Could you check a few things on this model? Use its own coordinates, in mm. Face numbers are marked on the shaded views. A direction names the side the tool comes from. Give positions to 0.01 mm unless a question says otherwise; leave off trailing zeros. Write each loop counter-clockwise with the first axis right and the second up, starting at its lowest first coordinate (ties: lowest second). Pieces come first, ordered by that corner, then holes. Notation, with made-up numbers: M -35.75,-24 L -16.75,-24 A18 cw -16.75,-11 Z; hole C 54.5,12 d2. An arc over 180 degrees is marked long. One line per item, written item: value.
```python
from build123d import *

# Parameters (mm, degrees)
F0_R      = 38.84
F0_R_2    = 27.5
F1_DEPTH  = 10.14
F2_R      = 41.875
F3_DEPTH  = 4.57
F4_R      = 41.875
F6_R      = 40.925
F8_R      = 40
F9_DEPTH  = 8.65
F10_R     = 41.95
F11_DEPTH = 13.57
F12_R     = 39.7
F13_DEPTH = 11.49
F14_R     = 31
F15_DEPTH = 16.29
F16_R     = 27.295707
F17_DEPTH = 2.75
F18_R     = 29.375
F19_DEPTH = 6
F20_R     = 28.5
F21_DEPTH = 1.3
F22_R     = 27.25
F23_DEPTH = 5.5
F24_R     = 28.475
F25_DEPTH = 12.25


with BuildPart() as f1:
    # F0 (on Front) → F1 (new body)
    with BuildSketch(Plane.XZ):
        Circle(F0_R)
        Circle(F0_R_2, mode=Mode.SUBTRACT)
    extrude(amount=F1_DEPTH)

    # F2 (on face) → F3 (join)
    with BuildSketch(Plane.XZ.offset(10.14)):
        Circle(F2_R)
    extrude(amount=F3_DEPTH)

    # F4 (on face) → F7 section 0
    with BuildSketch(Plane.XZ.offset(14.71)):
        Circle(F4_R)
    # F6 (on offset) → F7 section 1
    with BuildSketch(Plane.XZ.offset(19.21)):
        Circle(F6_R)
    loft()

    # F8 (on face) → F9 (join)
    with BuildSketch(Plane.XZ.offset(19.21)):
        Circle(F8_R)
    extrude(amount=F9_DEPTH)

    # F10 (on face) → F11 (join)
    with BuildSketch(Plane.XZ.offset(27.86)):
        Circle(F10_R)
    extrude(amount=F11_DEPTH)

    # F12 (on face) → F13 (cut)
    with BuildSketch(Plane.XZ.offset(41.43)):
        Circle(F12_R)
    extrude(amount=-F13_DEPTH, mode=Mode.SUBTRACT)

    # F14 (on face) → F15 (join)
    with BuildSketch(Plane.XZ.offset(29.94)):
        Circle(F14_R)
    extrude(amount=F15_DEPTH)

    # F16 (on face) → F17 (join)
    with BuildSketch(Plane.XZ.offset(46.23)):
        Circle(F16_R)
    extrude(amount=F17_DEPTH)

    # F18 (on face) → F19 (join)
    with BuildSketch(Plane.XZ.offset(48.98)):
        Circle(F18_R)
    extrude(amount=F19_DEPTH)

    # F20 (on face) → F21 (join)
    with BuildSketch(Plane.XZ.offset(54.98)):
        Circle(F20_R)
    extrude(amount=F21_DEPTH)

    # F22 (on face) → F23 (join)
    with BuildSketch(Plane.XZ.offset(56.28)):
        Circle(F22_R)
    extrude(amount=F23_DEPTH)

    # F24 (on face) → F25 (join)
    with BuildSketch(Plane.XZ.offset(61.78)):
        Circle(F24_R)
    extrude(amount=F25_DEPTH)


solid = f1.part
```
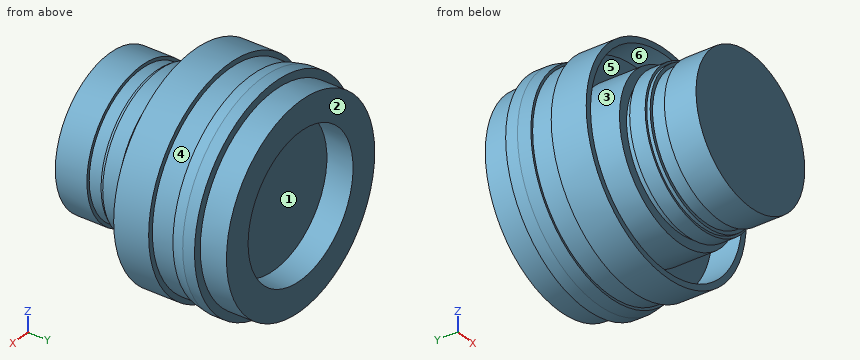
1) I'm going to push flat-ended pins straight in: pin 1 (5 mm diameter, centred on y = -37.5, z = 6, fed in from -X); pin 2 (12 mm diameter, centred on x = -0.5, y = -42.5, fed in from -Z); pin 3 (12 mm diameter, centred on y = -31.5, z = -14.5, fed in from -X); pin 4 (10 mm diameter, centred on y = -43, z = 3.5, fed in from +X). Where does each tip first touch, or does it pass through?
Outcome:
pin 1: stops at x = -41.8
pin 2: stops at z = -41.95
pin 3: stops at x = -41.08
pin 4: stops at x = 41.95
2) On a 3-axis mill with a long thin cutter (end or side, diameter ignored), from which of +Z, -Z, +X, -X, +Y, -Y can I reach the whole of each face in a straight line? I mean the marked faces 1, 2 and 3. Say none if no direction works.
Outcome:
face 1: +Y
face 2: +Z, -Z, +X, -X, +Y
face 3: -Y
3) Please list where these lines run through material, in increasing order: L1, parallel to Z at x = 0, y = -34; L2, parallel to Y at x = -17, z = 22; L3, parallel to Y at x = 24.5, z = -32. Write a range as from..to.
Outcome:
L1: z = -41.95..-39.7, -31..31, 39.7..41.95
L2: y = -74.03..-61.78, -56.28..-48.98, -46.23..0
L3: y = -41.43..-27.86, -19.21..-10.14
4) If we section it at C-C, the plane y = -44.5: Write out the boundary of the cut face in (x, z), then the cut area to 3 significant figures.
Outcome:
outline: C 0,0 d62
area: 3,020 mm^2
5) If we section it at A-A, the plane y = -5: Write out the boundary of the cut face in (x, z).
Outcome:
outline: C 0,0 d77.68; hole C 0,0 d55
6) If we section it at B-B, the plane y = -67: Write out the boundary of the cut face in (x, z) (3 decimals).
Outcome:
outline: C 0,0 d56.95
7) We'd pull the mould along Y, two halves only. Please class the marked faces 4, 5 and 6: pulls with the +Y half, pulls with the -Y half, needs draft (parallel to the pull), parting line crosses it, or undercut.
Outcome:
face 4: undercut
face 5: pulls with the -Y half
face 6: needs draft
